```python
from build123d import *

# Parameters (mm, degrees)
SKETCH1_W                 = 5.08
SKETCH1_H                 = 78.74
SKETCH1_W_2               = 21.59
SKETCH1_H_2               = 8.89
BOSS_EXTRUDE1_DEPTH       = 35.56
SKETCH2_R                 = 11.303
CUT_EXTRUDE1_DEPTH        = 4.953
F_8_CLEARANCE_HOLE1_D     = 4.9149
CUT_EXTRUDE4_REACH        = 91.054
SKETCH5_R                 = 7.747
F_6_CLEARANCE_HOLE1_D     = 4.3053
F_6_CLEARANCE_HOLE1_DEPTH = 5.08
BOSS_EXTRUDE3_DEPTH       = 13.3985
BOSS_EXTRUDE4_DEPTH       = 13.3985
SKETCH21_R                = 38.1
CUT_EXTRUDE5_DEPTH        = 91.420075758
SKETCH22_W                = 17.828699099
SKETCH22_H                = 30.684129503
CUT_EXTRUDE6_DEPTH        = 121.92


with BuildPart() as part:
    # Sketch1 → Boss-Extrude1 (new body)
    with BuildSketch(Plane(origin=(0, 0, 0), x_dir=(1, 0, 0), z_dir=(0, 1, 0))):
        with Locations((2.54, 39.37)):
            Rectangle(SKETCH1_W, SKETCH1_H)
        with Locations((15.875, 4.445)):
            Rectangle(SKETCH1_W_2, SKETCH1_H_2)
    extrude(amount=BOSS_EXTRUDE1_DEPTH)

    # Sketch2 → Cut-Extrude1 (cut)
    with BuildSketch(Plane.XY):
        with Locations((13.335, 17.78)):
            Circle(SKETCH2_R)
    extrude(amount=-CUT_EXTRUDE1_DEPTH, mode=Mode.SUBTRACT)

    # #8 Clearance Hole1 (through all)
    with Locations(Plane.XY.offset(-4.953)):
        with Locations((13.335, 17.78)):
            Hole(F_8_CLEARANCE_HOLE1_D / 2)

    # Sketch5 → Cut-Extrude4 (cut, up to next)
    with BuildSketch(Plane(origin=(5.08, 0, 0), x_dir=(0, 0, -1), z_dir=(1, 0, 0)), mode=Mode.PRIVATE) as cut_extrude4_sk1:
        with Locations((46.736, 17.78)):
            Circle(SKETCH5_R)
    cut_extrude4_tool1 = extrude(cut_extrude4_sk1.sketch, amount=-CUT_EXTRUDE4_REACH, mode=Mode.PRIVATE) & part.part
    # Sketch5 → Cut-Extrude4 (cut, up to next)
    with BuildSketch(Plane(origin=(5.08, 0, 0), x_dir=(0, 0, -1), z_dir=(1, 0, 0)), mode=Mode.PRIVATE) as cut_extrude4_sk2:
        with BuildLine():
            ThreePointArc((54.483, 17.78), (46.736, 25.527), (38.989, 17.78))
            Line((38.989, 17.78), (54.483, 17.78))
        make_face()
    cut_extrude4_tool2 = extrude(cut_extrude4_sk2.sketch, amount=-CUT_EXTRUDE4_REACH, mode=Mode.PRIVATE) & part.part
    # Sketch5 → Cut-Extrude4 (cut, up to next)
    with BuildSketch(Plane(origin=(5.08, 0, 0), x_dir=(0, 0, -1), z_dir=(1, 0, 0)), mode=Mode.PRIVATE) as cut_extrude4_sk3:
        with BuildLine():
            Line((54.483, 17.78), (38.989, 17.78))
            ThreePointArc((38.989, 17.78), (46.736, 10.033), (54.483, 17.78))
        make_face()
    cut_extrude4_tool3 = extrude(cut_extrude4_sk3.sketch, amount=-CUT_EXTRUDE4_REACH, mode=Mode.PRIVATE) & part.part
    add(cut_extrude4_tool1.solids().sort_by_distance((5.08, 17.78, -46.736))[0], mode=Mode.SUBTRACT)
    add(cut_extrude4_tool2.solids().sort_by_distance((5.08, 21.067929, -46.736))[0], mode=Mode.SUBTRACT)
    add(cut_extrude4_tool3.solids().sort_by_distance((5.08, 14.492071, -46.736))[0], mode=Mode.SUBTRACT)

    # #6 Clearance Hole1
    with Locations(Plane(origin=(5.08, 0, 0), x_dir=(0, 0, -1), z_dir=(1, 0, 0))):
        with Locations((34.544, 17.78), (46.736, 17.78), (64.516, 26.162), (64.516, 9.398)):
            Hole(F_6_CLEARANCE_HOLE1_D / 2, depth=F_6_CLEARANCE_HOLE1_DEPTH)

    # Sketch17 → Boss-Extrude3 (add)
    with BuildSketch(Plane(origin=(0, 35.56, 0), x_dir=(1, 0, 0), z_dir=(0, 1, 0))):
        Polygon((5.08, 8.89), (5.08, 34.29), (26.67, 8.89), align=None)
    extrude(amount=-BOSS_EXTRUDE3_DEPTH)

    # Sketch18 → Boss-Extrude4 (add)
    with BuildSketch(Plane.XZ):
        Polygon((26.67, -8.89), (5.08, -8.89), (5.08, -34.29), align=None)
    extrude(amount=-BOSS_EXTRUDE4_DEPTH)

    # Sketch21 → Cut-Extrude5 (cut, through all)
    with BuildSketch(Plane(origin=(0, 35.56, 0), x_dir=(1, 0, 0), z_dir=(0, 1, 0))):
        with Locations((44.937862921, 45.023006442)):
            Circle(SKETCH21_R)
    extrude(amount=-CUT_EXTRUDE5_DEPTH, mode=Mode.SUBTRACT)

    # Sketch22 → Cut-Extrude6 (cut)
    with BuildSketch(Plane(origin=(0, 35.56, 0), x_dir=(1, 0, 0), z_dir=(0, 1, 0))):
        with Locations((18.355186326, 24.356358653)):
            Rectangle(SKETCH22_W, SKETCH22_H)
    extrude(amount=-CUT_EXTRUDE6_DEPTH, mode=Mode.SUBTRACT)


solid = part.part
```
Read the model definition and answer for the solid it produces. Units are mm, in the model's axes. A direction names the side the tool comes from. Round coordinates to 2 decimals unless told otherwise and drop trailing zeros. Write each loop counter-clockwise with the first axis right and the second up, starting at its lowest first coordinate (ties: lowest second). Pieces come first, ordered by that corner, then holes. Notation, with made-up numbers: (-15.75, 81) -> (-3.75, 81) arc R33 cw to (-3.75, 117) -> close; hole circle Ø2 at (23, -16.75). An arc over 180 degrees is marked (long way). Answer in a Markdown table with one row per item. Add a question column.
1) Find section C-C, the plane z = -13.5. Determine the outline of the cut face in (x, y).
2) Find section D-D, the plane y = 8. Determine the outline of the cut face in (x, z), and give its area (3 significant figures).
3) Given P1, Ø6, axis at y = 27, z = -55, coming from the +X side; P2, Ø10.5, axis at x = 21.5, y = 26, coming from the -Z side; P3, Ø4, axis at y = 8.5, z = -16, coming from the +X side; P4, Ø3.5, axis at y = 9.398, z = -64.516, coming from the -X side, each flat-ended and moving along its own axis, determine where each tip first touches the part or whether it passes through.
4) Determine the mould class of faces 4 (the face through (26.67, 18, -4)), 5 (the face through (13, 6, 0)), 6 (the face through (3, 18, -78.74)), 7 (the face through (2.5, 10.04, -62.46)) for opening direction Z: pulls with the +Z half, pulls with the -Z half, needs draft (parallel to the pull), parting line crosses it, or undercut.
5) Find section B-B, the plane x = 12.5. Determine the outline of the cut face in (y, z).
6) Consider line 1 (Z direction, x = 25, y = 30.5); line 2 (Z direction, x = 9.75, y = 12); line 3 (X direction, y = 28.5, z = -44). Determine where each line is inside the solid, lowest interval first.
7) Which of the six approach directions +Z, -Z, +X, -X, +Y, -Y give full straight-line access (tool end or side, diameter ignored) to faces 1 (the face through (16, 19, -8.89)), 2 (the face through (18, 7, -9.014)), 3 (the face through (4, 0, -25))?
8) Find section A-A, the plane y = 17.78. Determine the outline of the cut face in (x, z), and give its area (3 significant figures).
Findings below:
| question | item | result |
|---|---|---|
| 1 | outline | (0, 0) -> (9.44, 0) -> (9.44, 13.4) -> (5.08, 13.4) -> (5.08, 22.16) -> (9.44, 22.16) -> (9.44, 35.56) -> (0, 35.56) -> close |
| 2 | outline | (0, -78.74) -> (5.08, -78.74) -> (5.08, -66.15) -> (0, -66.15) -> close; (0, -62.88) -> (5.08, -62.88) -> (5.08, -34.29) -> (9.44, -29.16) -> (9.44, -9.01) -> (26.56, -9.01) -> (26.67, -8.89) -> (26.67, 0) -> (19, 0) -> (19, -4.95) -> (7.67, -4.95) -> (7.67, 0) -> (0, 0) -> close |
| 2 | area | 621 mm² |
| 3 | P1 | x = 5.08 |
| 3 | P2 | z = -9.01 |
| 3 | P3 | x = 9.44 |
| 3 | P4 | through |
| 4 | face 4 | needs draft |
| 4 | face 5 | pulls with the +Z half |
| 4 | face 6 | pulls with the -Z half |
| 4 | face 7 | undercut |
| 5 | outline | (0, -9.01) -> (13.4, -9.01) -> (13.4, -8.89) -> (15.47, -8.89) -> (15.47, -4.95) -> (6.51, -4.95) -> (6.51, 0) -> (0, 0) -> close; (20.09, -8.89) -> (22.16, -8.89) -> (22.16, -9.01) -> (35.56, -9.01) -> (35.56, 0) -> (29.05, 0) -> (29.05, -4.95) -> (20.09, -4.95) -> close |
| 6 | line 1 | -9.01 to 0 |
| 6 | line 2 | -9.01 to -4.95 |
| 6 | line 3 | 0 to 5.08 |
| 7 | face 1 | -Z, +X |
| 7 | face 2 | -Z, +X, +Y, -Y |
| 7 | face 3 | +Z, -Z, +X, -X, -Y |
| 8 | outline | (0, -78.74) -> (5.08, -78.74) -> (5.08, -54.48) -> (0, -54.48) -> close; (0, -38.99) -> (5.08, -38.99) -> (5.08, -36.7) -> (0, -36.7) -> close; (0, -32.39) -> (5.08, -32.39) -> (5.08, -8.89) -> (10.88, -8.89) -> (10.88, -4.95) -> (2.03, -4.95) -> (2.03, 0) -> (0, 0) -> close; (15.79, -8.89) -> (26.67, -8.89) -> (26.67, 0) -> (24.64, 0) -> (24.64, -4.95) -> (15.79, -4.95) -> close |
| 8 | area | 360 mm² |
